```python
from build123d import *

# Parameters (mm, degrees)
F2_W     = 32.4015552178
F2_H     = 32.2648398578
F3_DEPTH = 25
F4_R     = 0.2


with BuildPart() as f1:
    # F0 (on Front) → F1 (revolve)
    with BuildSketch(Plane.XZ):
        Polygon((22.2295931596, 4.1953726299), (20.2295931596, 4.1953726299), (20.2295931596, 2.6953726299), (19.4795931596, 2.6953726299), (19.4795931596, 0.1953726299), (22.2295931596, 0.1953726299), align=None)
    revolve(axis=Axis((25.9795931596, 0, 0.8535729721), (0, 0, -1)))

    # F2 (on Front) → F3 (cut)
    with BuildSketch(Plane.XZ):
        with Locations((27.7060153894, 1.3981740922)):
            Rectangle(F2_W, F2_H)
    extrude(amount=-F3_DEPTH, mode=Mode.SUBTRACT)

    # F4
    f4_edges = [f1.edges().sort_by_distance(p)[0] for p in [
        (25.979593, -5.75, 4.195373),
        (25.979593, -3.75, 4.195373),
    ]]
    fillet(f4_edges, radius=F4_R)


solid = f1.part
```
Read the model definition and answer for the solid it produces. Units are mm, in the model's axes. A direction names the side the tool comes from. Give positions to 0.01 mm unless a question says otherwise; leave off trailing zeros. Loops run counter-clockwise (first coordinate to the right, second up) from the corner with the lowest first, then second, coordinate; pieces in that order, holes last.
Item 1: Find the intervals of material crossed by line 1 along Z through (x, y) = (21, -2.5); line 2 along X through (y, z) = (-1.25, 3.8); line 3 along X through (y, z) = (-1.5, 1), in increasing order.
Item 2: Each of these flat-tipped pins is pushed along its axis until it touches: pin 1 Ø1.5 at (x, z) = (25, 3) entering from -Y; pin 2 Ø1 at (x, y) = (27, -1.5) entering from +Z. Where does it stop, or does it pass through?
Item 3: The mould has two halves that part along X. Classify faces 3 (the cylindrical face through (26.06, -3.75, 2.12)), 4 (the flat face through (21, 0, 2)), 5 (the cylindrical face through (26.11, -5.75, 3.34)): released by +X, released by -X, zero draft, split by the parting line, or undercut.
Item 4: For faces 1 (the flat face through (26, -6, 2.695)), 2 (the flat face through (31, 0, 2)), determine the directions among +Z, -Z, +X, -X, +Y, -Y from which every point of the face is accessible in a straight line to the end or side of a thin tool.
Item 5: The part is cut by section A-A (z = 1.75). Write down the section's boundary in (x, y).
Taken from the geometry:
1. line 1: z = 0.2 to 4.19
1. line 2: x = 20.37 to 22.44, 29.52 to 31.59
1. line 3: x = 19.66 to 22.54, 29.42 to 32.3
2. pin 1: stops at y = -6.49
2. pin 2: passes through
3. face 3: undercut
3. face 4: zero draft
3. face 5: split by the parting line
4. face 1: +Z, -Y
4. face 2: +Z, -Z, +X, -X, +Y
5. outline: (19.48, 0) arc R6.5 ccw to (32.48, 0) - (29.73, 0) arc R3.75 cw to (22.23, 0) - close
